```python
from build123d import *

# Parameters (mm, degrees)
F1_DEPTH = 6


with BuildPart() as f1:
    # F0 (on Front) → F1 (new body)
    with BuildSketch(Plane.XZ):
        with BuildLine():
            Line((43.369441, -58.054813), (53.369441, -58.054813))
            ThreePointArc((53.369441, -58.054813), (64.76999, -49.455363), (73.369441, -38.054813))
            Line((73.369441, -38.054813), (73.369441, -28.054813))
            Line((73.369441, -28.054813), (79.369441, -28.054813))
            Line((79.369441, -28.054813), (79.369441, -18.054813))
            Line((79.369441, -18.054813), (73.369441, -18.054813))
            Line((73.369441, -18.054813), (73.369441, -8.054813))
            Line((73.369441, -8.054813), (79.369441, -8.054813))
            Line((79.369441, -8.054813), (79.369441, 1.945187))
            Line((79.369441, 1.945187), (73.369441, 1.945187))
            Line((73.369441, 1.945187), (73.369441, 11.945187))
            ThreePointArc((73.369441, 11.945187), (64.76999, 23.345736), (53.369441, 31.945187))
            Line((53.369441, 31.945187), (43.369441, 31.945187))
            Line((43.369441, 31.945187), (43.369441, 37.945187))
            Line((43.369441, 37.945187), (33.369441, 37.945187))
            Line((33.369441, 37.945187), (33.369441, 31.945187))
            Line((33.369441, 31.945187), (23.369441, 31.945187))
            Line((23.369441, 31.945187), (23.369441, 37.945187))
            Line((23.369441, 37.945187), (13.369441, 37.945187))
            Line((13.369441, 37.945187), (13.369441, 31.945187))
            Line((13.369441, 31.945187), (3.369441, 31.945187))
            ThreePointArc((3.369441, 31.945187), (-8.031109, 23.345736), (-16.630559, 11.945187))
            Line((-16.630559, 11.945187), (-16.630559, 0.945187))
            Line((-16.630559, 0.945187), (-22.630559, 0.945187))
            Line((-22.630559, 0.945187), (-22.630559, 6.945187))
            Line((-22.630559, 6.945187), (-42.630559, 6.945187))
            Line((-42.630559, 6.945187), (-42.630559, 0.945187))
            Line((-42.630559, 0.945187), (-62.630559, 0.945187))
            Line((-62.630559, 0.945187), (-62.630559, -27.054813))
            Line((-62.630559, -27.054813), (-42.630559, -27.054813))
            Line((-42.630559, -27.054813), (-42.630559, -33.054813))
            Line((-42.630559, -33.054813), (-22.630559, -33.054813))
            Line((-22.630559, -33.054813), (-22.630559, -27.054813))
            Line((-22.630559, -27.054813), (-16.630559, -27.054813))
            Line((-16.630559, -27.054813), (-16.630559, -38.054813))
            ThreePointArc((-16.630559, -38.054813), (-8.031109, -49.455363), (3.369441, -58.054813))
            Line((3.369441, -58.054813), (13.369441, -58.054813))
            Line((13.369441, -58.054813), (13.369441, -64.054813))
            Line((13.369441, -64.054813), (23.369441, -64.054813))
            Line((23.369441, -64.054813), (23.369441, -58.054813))
            Line((23.369441, -58.054813), (33.369441, -58.054813))
            Line((33.369441, -58.054813), (33.369441, -64.054813))
            Line((33.369441, -64.054813), (43.369441, -64.054813))
            Line((43.369441, -64.054813), (43.369441, -58.054813))
        make_face()
    extrude(amount=F1_DEPTH)


solid = f1.part
```
Work out the finished part from the listing and answer in its coordinate system (mm). A direction names the side the tool comes from. Give positions to 0.01 mm unless a question says otherwise; leave off trailing zeros. Order: outer loops, then holes, each group sorted by start corner. A loop starts at its lowest first (then second) coordinate and runs counter-clockwise, first axis right, second up. Notation, with made-up numbers: M 0,30 L 55,30 A29 cw 55,56 Z; hole C 85,69.5 d2. An arc over 180 degrees is marked long. Return JSON: item names as keys, results as strings.
1) Section B-B, the plane x = 10 is taken. Write down the section's boundary in (y, z).
Resolved:
{"outline": "M -6,-58.05 L 0,-58.05 L 0,31.95 L -6,31.95 Z"}
2) A tool of negligible diameter and unlimited length cuts with its end or side. For faces 5 (the flat face through (-32, -3, 6.945)), 6 (the flat face through (76, -3, -8.055)), 7 (the flat face through (8, -3, -58.055)), 8 (the flat face through (76, -3, -28.055)), 9 (the flat face through (23.369, -3, -61)), from which of +Z, -Z, +X, -X, +Y, -Y can it reach the whole face along a straight path? Write none if from no direction.
Resolved:
{"face 5": "+Z, -X, +Y, -Y", "face 6": "+X, +Y, -Y", "face 7": "-Z, -X, +Y, -Y", "face 8": "-Z, +X, +Y, -Y", "face 9": "-Z, +Y, -Y"}
3) Section A-A, the plane z = -36 is taken. Write down the section's boundary in (x, y).
Resolved:
{"outline": "M -16.63,-6 L 73.37,-6 L 73.37,0 L -16.63,0 Z"}
4) For a pull along X with two mould halves and no side action, classify faces 1 (the flat face through (43.369, -3, 35)), 2 (the flat face through (38, -3, -64.055)), 3 (the flat face through (28, -3, 31.945)), 4 (the flat face through (-22.631, -3, -30)) as +X half, -X half, draft (parallel to the pull), parting line (faces both ways), or undercut.
Resolved:
{"face 1": "+X half", "face 2": "draft", "face 3": "undercut", "face 4": "undercut"}
5) Each of these flat-tipped pins is pushed along its axis until it touches: pin 1 (1 mm diameter, centred on y = -4.5, z = 22, fed in from +X); pin 2 (3 mm diameter, centred on x = 77, y = -3.5, fed in from +Z); pin 3 (3 mm diameter, centred on y = -2.5, z = -60.5, fed in from -X). Where does it stop, or does it pass through?
Resolved:
{"pin 1": "x = 66.53", "pin 2": "z = 1.95", "pin 3": "x = 13.37"}
6) Straight lines are drawn through the part: line 1 along Z through (x, y) = (-49, -5.1); line 2 along Z through (x, y) = (4, -1); line 3 along X through (y, z) = (-0.3, 11.5). For each, find the intervals that lie inside material, in ascending order. Write a range as [from, to].
Resolved:
{"line 1": "[-27.05, 0.95]", "line 2": "[-58.05, 31.95]", "line 3": "[-16.63, 73.37]"}
